```python
from build123d import *

# Parameters (mm, degrees)
SKETCH1_R           = 50.8
BOSS_EXTRUDE1_DEPTH = 457.2
SKETCH2_R           = 41.275
CUT_EXTRUDE1_DEPTH  = 457.2
SKETCH3_R           = 66.675
BOSS_EXTRUDE2_DEPTH = 6.35


with BuildPart() as part:
    # Sketch1 → Boss-Extrude1 (new body)
    with BuildSketch(Plane.XY):
        Circle(SKETCH1_R)
    extrude(amount=BOSS_EXTRUDE1_DEPTH)

    # Sketch2 → Cut-Extrude1 (cut)
    with BuildSketch(Plane.XY.offset(457.2)):
        Circle(SKETCH2_R)
    extrude(amount=-CUT_EXTRUDE1_DEPTH, mode=Mode.SUBTRACT)

    # Sketch3 → Boss-Extrude2 (add)
    with BuildSketch(Plane.XY.offset(457.2)):
        Circle(SKETCH3_R)
    boss_extrude2 = extrude(amount=BOSS_EXTRUDE2_DEPTH)

    # Mirror1: Boss-Extrude2 across plane
    add(boss_extrude2.mirror(Plane.XY.offset(228.6)))


solid = part.part
```
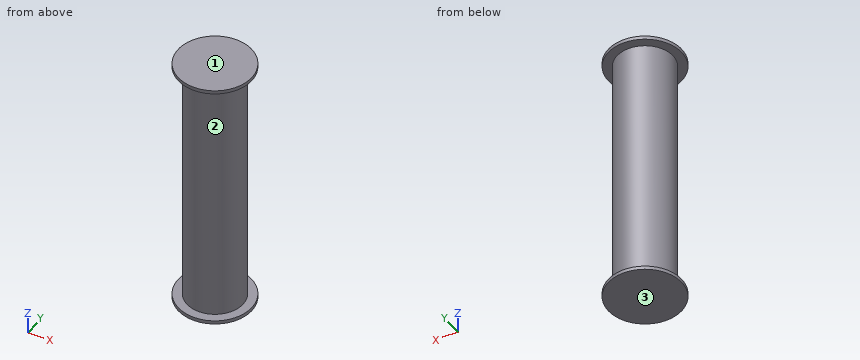
The listing builds one solid part. Answer for the finished solid, in the listing's coordinates (mm). Face numbers are marked on the shaded views. Coordinates: 2 decimals unless noted, no trailing zeros. Write each loop counter-clockwise with the first axis right and the second up, starting at its lowest first coordinate (ties: lowest second). Pieces come first, ordered by that corner, then holes. Notation, with made-up numbers: M 80.25,-14 L 86.25,-14 A19 cw 86.25,-10 Z; hole C 38,71 d4. An arc over 180 degrees is marked long. Use a Markdown table: item, result. Add a question column.
1. Section A-A (y = 0) is taken. Give the vertices of the cut face in (x, z) (3 decimals), plus the area to 3 significant figures.
2. Section D-D (z = 140.5) is taken. Give the vertices of the cut face in (x, y) (3 decimals), plus the area to 3 significant figures.
3. Section C-C (y = 59.5) is taken. Give the vertices of the cut face in (x, z).
4. For a pull along Z with two mould halves and no side action, classify the marked faces 1, 2 and 3 as +Z half, -Z half, draft (parallel to the pull), parting line (faces both ways), or undercut.
5. Straight lines are drawn through the part: line 1 along Y through (x, z) = (0, 323) (3 decimals); line 2 along Z through (x, y) = (-17.5, -32); line 3 along Y through (x, z) = (35.5, 305.5). For each, find the intervals that lie inside material, in ascending order. Write a range as [from, to].
6. Given P1, Ø2, axis at y = -7, z = 80, coming from the -X side; P2, Ø1, axis at y = -41, z = 235.5, coming from the +X side; P3, Ø5, axis at x = 45.5, z = 185, coming from the -Y side, each flat-ended and moving along its own axis, determine where each tip first touches the part or whether it passes through.
Data:
| question | item | result |
|---|---|---|
| 1 | outline | M -66.675,-6.35 L 66.675,-6.35 L 66.675,0 L 50.8,0 L 50.8,457.2 L 66.675,457.2 L 66.675,463.55 L -66.675,463.55 L -66.675,457.2 L -50.8,457.2 L -50.8,0 L -66.675,0 Z; hole M -41.275,0 L 41.275,0 L 41.275,457.2 L -41.275,457.2 Z |
| 1 | area | 10,400 mm2 |
| 2 | outline | C 0,0 d101.6; hole C 0,0 d82.55 |
| 2 | area | 2,760 mm2 |
| 3 | outline | M -30.09,-6.35 L 30.09,-6.35 L 30.09,0 L -30.09,0 Z; M -30.09,457.2 L 30.09,457.2 L 30.09,463.55 L -30.09,463.55 Z |
| 4 | face 1 | +Z half |
| 4 | face 2 | undercut |
| 4 | face 3 | -Z half |
| 5 | line 1 | y = [-50.8, -41.275], [41.275, 50.8] |
| 5 | line 2 | z = [-6.35, 0], [457.2, 463.55] |
| 5 | line 3 | y = [-36.34, -21.06], [21.06, 36.34] |
| 6 | P1 | stops at x = -50.44 |
| 6 | P2 | stops at x = 30.67 |
| 6 | P3 | stops at y = -27.05 |
